```python
from build123d import *

# Parameters (mm, degrees)
F1_DEPTH = 3
F2_R     = 2


with BuildPart() as f1:
    # F0 (on Top) → F1 (new body)
    with BuildSketch(Plane.XY):
        with BuildLine():
            ThreePointArc((10, 8), (9.4142135624, 9.4142135624), (8, 10))
            Line((8, 10), (-8, 10))
            ThreePointArc((-8, 10), (-9.4142135624, 9.4142135624), (-10, 8))
            Line((-10, 8), (-10, -8))
            ThreePointArc((-10, -8), (-9.4142135624, -9.4142135624), (-8, -10))
            Line((-8, -10), (8, -10))
            ThreePointArc((8, -10), (9.4142135624, -9.4142135624), (10, -8))
            Line((10, -8), (10, 8))
        make_face()
    extrude(amount=F1_DEPTH)

    # F2
    f2_edges = [f1.edges().sort_by_distance(p)[0] for p in [
        (-9.414214, 9.414214, 3),
    ]]
    fillet(f2_edges, radius=F2_R)


solid = f1.part
```
For this review, take the finished solid that the model builds, in its own axes (mm). Give positions to 0.01 mm unless a question says otherwise; leave off trailing zeros. Write each loop counter-clockwise with the first axis right and the second up, starting at its lowest first coordinate (ties: lowest second). Pieces come first, ordered by that corner, then holes. Notation, with made-up numbers: M 62,80 L 114,80 A26 ccw 114,113 Z; hole C 79,62 d4. An arc over 180 degrees is marked long. Answer as a JSON object with one key per item and string values. Group by question number.
Item 1: Consider section B-B on x = -6.75. Write out the cut boundary in (y, z).
Item 2: Consider section A-A on z = 2.2. Write out the cut boundary in (x, y).
Item 3: For probe 1 along Y at (x, z) = (-8.25, 1.5); probe 2 along X at (y, z) = (-1.25, 1.85); probe 3 along Z at (x, y) = (-3.75, 8.25), list the stretches that pass through material, from the lowest coordinate up. Write a range as [from, to].
Item 4: For pin 1 Ø2 at (x, y) = (1.5, -3) entering from -Z, flat-tipped, find the tip position at first contact; note if it passes through.
Check result:
{
 "1": {"outline": "M -10,0 L 10,0 L 10,1 A2 ccw 8,3 L -8,3 A2 ccw -10,1 Z"},
 "2": {"outline": "M -9.6,-8 A1.6 ccw -8,-9.6 L 8,-9.6 A1.6 ccw 9.6,-8 L 9.6,8 A1.6 ccw 8,9.6 L -8,9.6 A1.6 ccw -9.6,8 Z"},
 "3": {"probe 1": "y = [-9.92, 9.92]", "probe 2": "x = [-9.81, 9.81]", "probe 3": "z = [0, 2.98]"},
 "4": {"pin 1": "stops at z = 0"}
}
